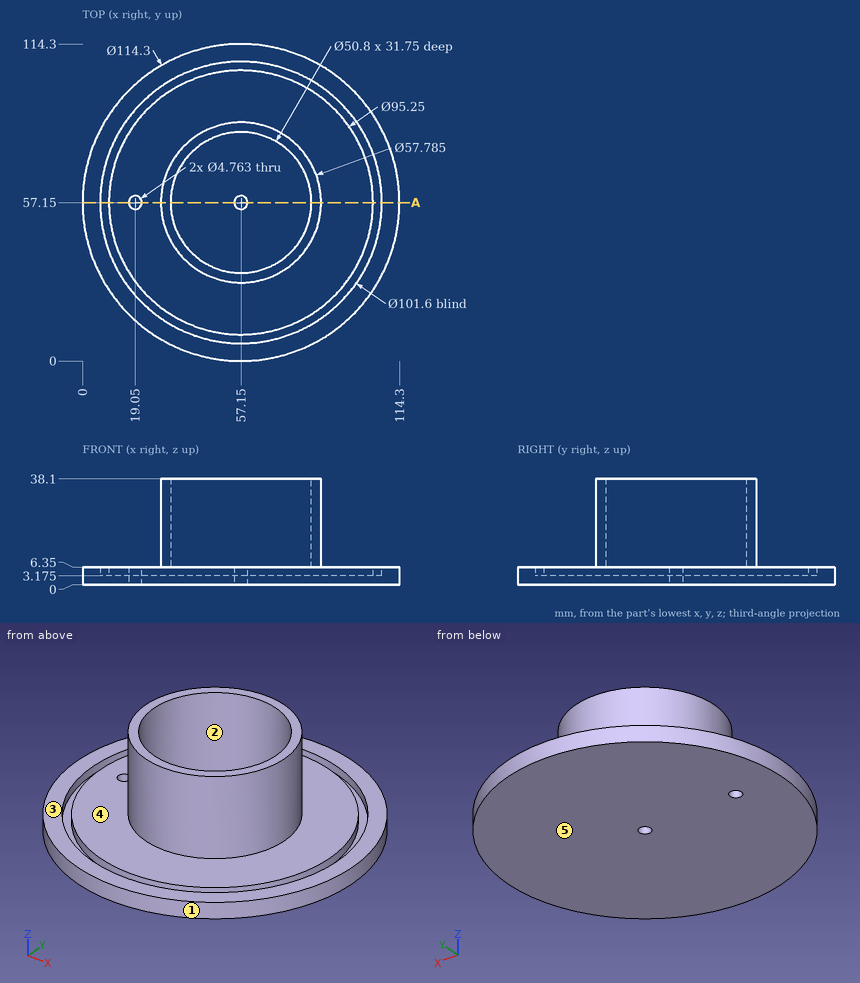
For this review, use the dimensioned drawing (mm, ordinates from the lowest corner) and the shaded views. A direction names the side the tool comes from. Give positions to 0.01 mm unless a question says otherwise; leave off trailing zeros.
Item 1: Insertion check: pin 1 (8 mm diameter, centred on x = 79, z = 12, fed in from +Y); pin 2 (10 mm diameter, centred on x = 57.5, z = 30, fed in from -Y); pin 3 (6 mm diameter, centred on x = 57.15, y = 57.15, fed in from +Z); pin 4 (2 mm diameter, centred on x = 14.5, y = 15, fed in from -Z). Each pin has a flat end and moves straight along its axis. Give the tip position at first contact, or say it passes through.
Item 2: Take a section at A-A, the plane y = 57.15. Give the number of separate pieces and of enclosed holes in the cut face, and give its area (3 significant figures).
Item 3: For line 1 along X through (y, z) = (57, 2); line 2 along Y through (x, z) = (57.15, 29.5); line 3 along Z through (x, y) = (94.5, 38.5), list the stretches that pass through material, from the lowest coordinate up.
Item 4: Draft analysis for pull direction X (two halves, no side actions). For the marked faces 1, 2 and 3, state which applies: +X half, -X half, draft (parallel to the pull), parting line (faces both ways), or undercut.
Item 5: Tool access review of the marked faces 4 and 5: name each direction out of +Z, -Z, +X, -X, +Y, -Y from which nothing blocks a thin tool from reaching the whole face with its end or side.
Calculated:
1. pin 1: stops at y = 79.87
1. pin 2: stops at y = 28.26
1. pin 3: stops at z = 6.35
1. pin 4: passes through
2. separate pieces: 3
2. enclosed holes: 0
2. area: 867 mm2
3. line 1: x = 0 to 16.67, 21.43 to 54.77, 59.53 to 114.3
3. line 2: y = 28.26 to 31.75, 82.55 to 86.04
3. line 3: z = 0 to 6.35
4. face 1: parting line
4. face 2: undercut
4. face 3: draft
5. face 4: +Z
5. face 5: -Z, +X, -X, +Y, -Y
